Model file for the job. Use its own axes, mm. A direction names the side the tool comes from. Give positions to 0.01 mm unless a question says otherwise; leave off trailing zeros. Order: outer loops, then holes, each group sorted by start corner. A loop starts at its lowest first (then second) coordinate and runs counter-clockwise, first axis right, second up. Notation, with made-up numbers: M 20,30 L 61,30 A16 cw 61,50 Z; hole C 64.5,27 d4. An arc over 180 degrees is marked long. Return JSON: item names as keys, results as strings. Group by question number.
1. Two-plate mould, pull along Z, no slides. Class faces 3 (the face through (13, -21, -5)), 4 (the face through (0.493, -1.947, -2.539)), 5 (the face through (0.044, 5.452, -17.312)): released by +Z, released by -Z, zero draft, split by the parting line, or undercut.
2. Slice it at A-A on z = 0. List the corners of the cut face in (x, y), then the cut area to 3 significant figures.
3. Pin check, flat tips, straight feed: pin 1 (4 mm diameter, centred on x = 4.5, y = -3, fed in from +Z); pin 2 (4 mm diameter, centred on y = 11.5, z = 3, fed in from +X); pin 3 (1.5 mm diameter, centred on y = 0, z = -0.5, fed in from -X); pin 4 (1.5 mm diameter, centred on x = 7, z = 3, fed in from -Y). Stop position of each tip, or through.
4. 3-axis set-ups, long thin cutter, end or side, ignore diameter. For faces 1 (the face through (6.77, 6.58, -20.89)), 2 (the face through (1, 0, -4)): which of +Z, -Z, +X, -X, +Y, -Y reach the whole face in a straight line?
5. Wall check: probe 1 along Y at (x, z) = (5.25, -0.5); probe 2 along Y at (x, z) = (0.8, 0); probe 3 along X at (y, z) = (11, -3.5). Give the ranges that are in metal, low to high. Write a range as [from, to].
6. Slice it at C-C on x = 7.5. List the corners of the cut face in (y, z).
from build123d import *

# Parameters (mm, degrees)
SKETCH1_R           = 21.9
BOSS_EXTRUDE1_DEPTH = 1
SKETCH2_R           = 21.9
SKETCH2_R_2         = 21.4
BOSS_EXTRUDE2_DEPTH = 12
SKETCH3_R           = 3.2
CUT_EXTRUDE1_DEPTH  = 12
CHAMFER1_SIZE       = 4
CHAMFER1_SIZE2      = 0.705307923


with BuildPart() as part:
    # Sketch1 → Boss-Extrude1 (new body)
    with BuildSketch(Plane.YZ):
        with Locations(Location((0, 0, 0), (0, 0, 270))):
            Circle(SKETCH1_R)
    extrude(amount=BOSS_EXTRUDE1_DEPTH)

    # Sketch2 → Boss-Extrude2 (add)
    with BuildSketch(Plane.YZ.offset(1)):
        with Locations(Location((0, 0, 0), (0, 0, 270))):
            Circle(SKETCH2_R)
        with Locations(Location((0, 0, 0), (0, 0, 270))):
            Circle(SKETCH2_R_2, mode=Mode.SUBTRACT)
    extrude(amount=BOSS_EXTRUDE2_DEPTH)

    # Sketch3 → Cut-Extrude1 (cut)
    with BuildSketch(Plane(origin=(0, 0, 0), x_dir=(0, -1, 0), z_dir=(-1, 0, 0))):
        with Locations(Location((0, 0, 0), (0, 0, 90))):
            Circle(SKETCH3_R)
    extrude(amount=-CUT_EXTRUDE1_DEPTH, mode=Mode.SUBTRACT)

    # Chamfer1
    chamfer1_edges = [part.edges().sort_by_distance(p)[0] for p in [
        (0, 0, 21.9),
    ]]
    chamfer1_side = [part.faces().sort_by_distance(p)[0] for p in [
        (0, 0, 21.28057446),
    ]]
    chamfer(chamfer1_edges, length=CHAMFER1_SIZE, length2=CHAMFER1_SIZE2, reference=chamfer1_side[0])


solid = part.part
Result:
{
 "1": {"face 3": "zero draft", "face 4": "undercut", "face 5": "split by the parting line"},
 "2": {"outline": "M 0,-17.9 L 0.71,-21.9 L 13,-21.9 L 13,-21.4 L 1,-21.4 L 1,-3.2 L 0,-3.2 Z; M 0,3.2 L 1,3.2 L 1,21.4 L 13,21.4 L 13,21.9 L 0.71,21.9 L 0,17.9 Z", "area": "46.6 mm2"},
 "3": {"pin 1": "stops at z = 21.88", "pin 2": "stops at x = 1", "pin 3": "passes through", "pin 4": "stops at y = -21.78"},
 "4": {"face 1": "+X, -X", "face 2": "+X"},
 "5": {"probe 1": "y = [-21.89, -21.39], [21.39, 21.89]", "probe 2": "y = [-21.9, -3.2], [3.2, 21.9]", "probe 3": "x = [0, 1]"},
 "6": {"outline": "C 0,0 d43.8; hole C 0,0 d42.8"}
}
